Read the model definition and answer for the solid it produces. Units are mm, in the model's axes. Face numbers are marked on the shaded views. A direction names the side the tool comes from. Give positions to 0.01 mm unless a question says otherwise; leave off trailing zeros. Order: outer loops, then holes, each group sorted by start corner. A loop starts at its lowest first (then second) coordinate and runs counter-clockwise, first axis right, second up. Notation, with made-up numbers: (11, -16.75) - (70, -16.75) arc R18 cw to (70, -5.75) - close; hole circle Ø3 at (18, 68). An arc over 180 degrees is marked (long way). Write each question's results on one line, items separated by ' | '.
from build123d import *

# Parameters (mm, degrees)
SKETCH1_W           = 30
SKETCH1_H           = 40
BOSS_EXTRUDE1_DEPTH = 13
SKETCH2_R           = 2.38125
CUT_EXTRUDE1_DEPTH  = 39.327535793
SKETCH3_R           = 2.8067
CUT_EXTRUDE2_DEPTH  = 10
FILLET1_R           = 7.5


with BuildPart() as part:
    # Sketch1 → Boss-Extrude1 (new, symmetric)
    with BuildSketch(Plane(origin=(0, 0, 0), x_dir=(0, 0, -1), z_dir=(1, 0, 0))):
        Rectangle(SKETCH1_W, SKETCH1_H)
    extrude(amount=BOSS_EXTRUDE1_DEPTH, both=True)

    # Sketch2 → Cut-Extrude1 (cut, through all)
    with BuildSketch(Plane.XY.offset(15)):
        with BuildLine():
            Line((-13, 20), (-13, -10))
            Line((-13, -10), (-4.775007753, 16.483004032))
            ThreePointArc((-4.775007753, 16.483004032), (-2.965213301, 19.025855198), (0, 20))
            Line((0, 20), (-13, 20))
        make_face()
        with Locations((0, 15)):
            Circle(SKETCH2_R)
        with BuildLine():
            Line((13, 20), (0, 20))
            ThreePointArc((0, 20), (2.965213301, 19.025855198), (4.775007753, 16.483004032))
            Line((4.775007753, 16.483004032), (13, -10))
            Line((13, -10), (13, 20))
        make_face()
    extrude(amount=-CUT_EXTRUDE1_DEPTH, mode=Mode.SUBTRACT)

    # Sketch3 → Cut-Extrude2 (cut)
    with BuildSketch(Plane.XZ.offset(20)):
        with Locations(Location((0, 10, 0), (0, 0, 270))):
            Circle(SKETCH3_R)
        with Locations(Location((0, -10, 0), (0, 0, 270))):
            Circle(SKETCH3_R)
        with Locations(Location((-10, 0, 0), (0, 0, 270))):
            Circle(SKETCH3_R)
        with Locations(Location((10, 0, 0), (0, 0, 270))):
            Circle(SKETCH3_R)
    extrude(amount=-CUT_EXTRUDE2_DEPTH, mode=Mode.SUBTRACT)

    # Fillet1
    fillet1_edges = [part.edges().sort_by_distance(p)[0] for p in [
        (-13, -15, 15),
        (13, -15, 15),
        (13, -15, -15),
        (-13, -15, -15),
    ]]
    fillet(fillet1_edges, radius=FILLET1_R)


solid = part.part
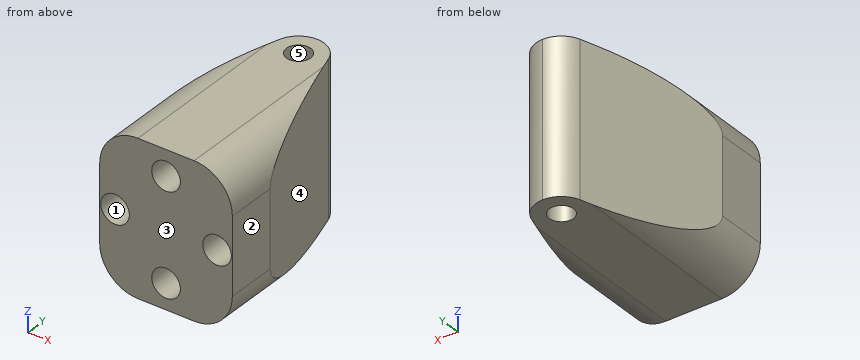
(1) Consider probe 1 along X at (y, z) = (-14.5, 0); probe 2 along Z at (x, y) = (1, -16.5); probe 3 along Y at (x, z) = (0.5, -11). Determine where each line is inside the solid, lowest interval first. Write a range as [from, to].
Conclusion:
probe 1: [-13, -12.81], [-7.19, 7.19], [12.81, 13] | probe 2: [-15, -12.62], [-7.38, 7.38], [12.62, 15] | probe 3: [-10, 12.67], [17.33, 19.97]
(2) For the marked faces 1 and 2, determine the directions among +Z, -Z, +X, -X, +Y, -Y from which every point of the face is accessible in a straight line to the end or side of a thin tool.
Conclusion:
face 1: -Y | face 2: +Z, -Z, +X, +Y, -Y
(3) Section A-A (z = 4) is taken. Give the vertices of the cut face in (x, y) (1 decimal).
Conclusion:
outline: (-13, -20) - (13, -20) - (13, -10) - (4.8, 16.5) arc R5 ccw to (-4.8, 16.5) - (-13, -10) - close; hole circle Ø4.8 at (0, 15)
(4) Section B-B (y = 15) is taken. Give the vertices of the cut face in (x, z).
Conclusion:
outline: (-5.24, -15) - (-2.38, -15) - (-2.38, 15) - (-5.24, 15) - close; (2.38, -15) - (5.24, -15) - (5.24, 15) - (2.38, 15) - close
(5) Each of these flat-tipped pins is pushed along its axis until it touches: pin 1 (4.5 mm diameter, centred on x = 1, z = 9, fed in from -Y); pin 2 (1.5 mm diameter, centred on y = 10, z = -4, fed in from -X); pin 3 (3.5 mm diameter, centred on x = 0, z = -10, fed in from -Y); pin 4 (2 mm diameter, centred on x = -1.5, z = -10.5, fed in from +Y). Where does it stop, or does it pass through?
Conclusion:
pin 1: y = -20 | pin 2: x = -7.02 | pin 3: y = -10 | pin 4: y = 19.97
(6) Section C-C (x = 10) is taken. Give the vertices of the cut face in (y, z).
Conclusion:
outline: (-20, -13.5) - (-0.34, -13.5) - (-0.34, 13.5) - (-20, 13.5) - (-20, 2.81) - (-10, 2.81) - (-10, -2.81) - (-20, -2.81) - close
(7) The mould has two halves that part along X. Classify the marked faces 3, 4 and 5: pulls with the +X half, pulls with the -X half, needs draft (parallel to the pull), parting line crosses it, or undercut.
Conclusion:
face 3: needs draft | face 4: pulls with the +X half | face 5: undercut
